Answer from the drawing. Dimensions are ordinates in mm from the lowest x, y and z of the part. A direction names the side the tool comes from. Round coordinates to 2 decimals unless told otherwise and drop trailing zeros. Write each loop counter-clockwise with the first axis right and the second up, starting at its lowest first coordinate (ties: lowest second). Pieces come first, ordered by that corner, then holes. Notation, with made-up numbers: (-24, 76.25) - (-9, 76.25) arc R25 cw to (-9, 98.25) - close; hole circle Ø2 at (28.25, 81). An arc over 180 degrees is marked (long way). Answer as a JSON object with one key per item and string values.
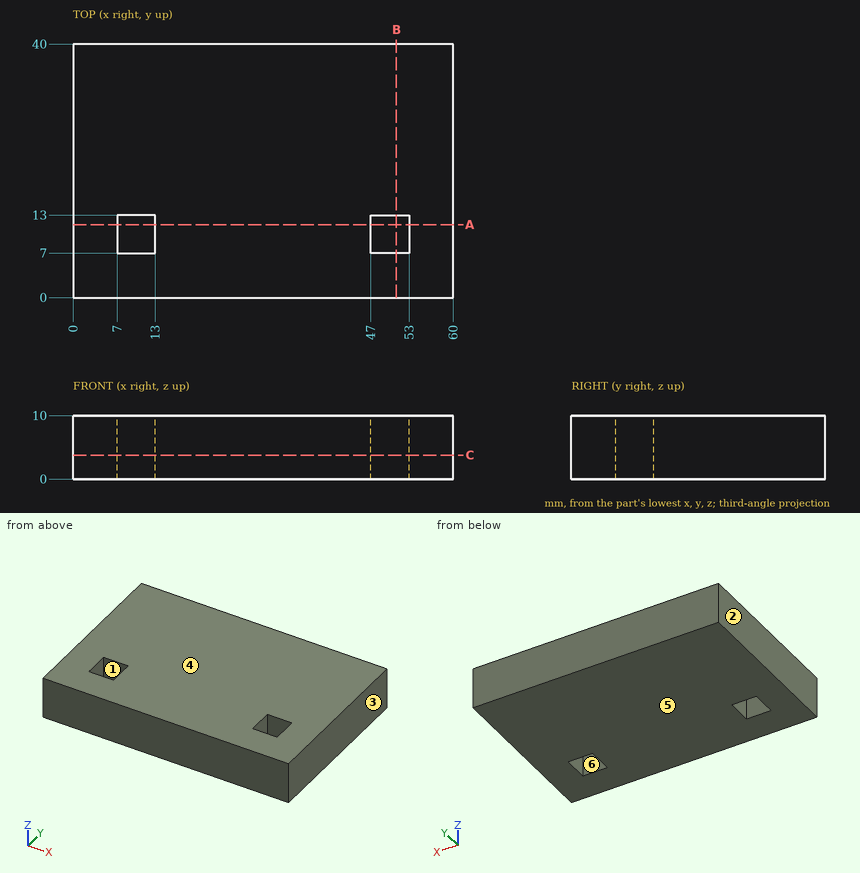
Item 1: Consider line 1 along X through (y, z) = (12.5, 7); line 2 along Y through (x, z) = (52, 7). Determine where each line is inside the solid, lowest interval first.
Results found:
{"line 1": "0 to 7, 13 to 47, 53 to 60", "line 2": "0 to 7, 13 to 40"}
Item 2: For the marked faces 5 and 6, determine the directions among +Z, -Z, +X, -X, +Y, -Y from which every point of the face is accessible in a straight line to the end or side of a thin tool.
Results found:
{"face 5": "-Z, +X, -X, +Y, -Y", "face 6": "+Z, -Z"}
Item 3: Determine the mould class of the marked faces 1, 2, 3 and 4 for opening direction X: pulls with the +X half, pulls with the -X half, needs draft (parallel to the pull), parting line crosses it, or undercut.
Results found:
{"face 1": "undercut", "face 2": "pulls with the -X half", "face 3": "pulls with the +X half", "face 4": "needs draft"}
Item 4: A cutting plane is placed at B-B (x = 51). Write down the section's boundary in (y, z).
Results found:
{"outline": "(0, 0) - (7, 0) - (7, 10) - (0, 10) - close; (13, 0) - (40, 0) - (40, 10) - (13, 10) - close"}
Item 5: A cutting plane is placed at C-C (z = 3.75). Write down the section's boundary in (x, y).
Results found:
{"outline": "(0, 0) - (60, 0) - (60, 40) - (0, 40) - close; hole (7, 7) - (13, 7) - (13, 13) - (7, 13) - close; hole (47, 7) - (53, 7) - (53, 13) - (47, 13) - close"}
Item 6: A cutting plane is placed at A-A (y = 11.5). Write down the section's boundary in (x, z).
Results found:
{"outline": "(0, 0) - (7, 0) - (7, 10) - (0, 10) - close; (13, 0) - (47, 0) - (47, 10) - (13, 10) - close; (53, 0) - (60, 0) - (60, 10) - (53, 10) - close"}
